Here's how the part is built. I have some questions about the finished solid (model axes, mm). A direction names the side the tool comes from. Coordinates: 2 decimals unless noted, no trailing zeros. Write each loop counter-clockwise with the first axis right and the second up, starting at its lowest first coordinate (ties: lowest second). Pieces come first, ordered by that corner, then holes. Notation, with made-up numbers: (-6.75, 53) -> (15.25, 53) arc R28 cw to (15.25, 92) -> close; hole circle Ø7 at (33.25, -23). An arc over 180 degrees is marked (long way). Use a Markdown table: item, result. Add a question column.
Item 1: On a 3-axis mill with a long thin cutter (end or side, diameter ignored), from which of +Z, -Z, +X, -X, +Y, -Y can I reach the whole of each face in a straight line? I mean faces 1 (the flat face through (0, 5, -12)), 2 (the flat face through (14.625, -3.5, -4)), 3 (the flat face through (0, 4, -26)), 4 (the cylindrical face through (0, -4, 1)). Say none if no direction works.
Item 2: Imagine slicing it at A-A, the plane x = 0. Write out the boundary of the cut face in (y, z), and give its area (3 significant figures).
Item 3: Will these pins go through, and if not, where does the flat tip stop? pin 1 Ø3 at (x, z) = (12, -16.5) entering from +Y; pin 2 Ø1 at (y, z) = (-6, -12) entering from +X (3 decimals); pin 3 Ø3 at (x, z) = (13.5, -14) entering from +Y.
Item 4: If we mould it in two halves opening along X, with no side actions, what happens to faces 5 (the flat face through (1, -5, 0)), 6 (the cylindrical face through (8.285, -2.699, -12.297)), 7 (the flat face through (-8, 2, -12))? For each: pulls with the +X half, pulls with the -X half, needs draft (parallel to the pull), parting line crosses it, or undercut.
Item 5: Imagine slicing it at C-C, the plane z = -4. Count the separate pieces of the cut face and the enclosed holes in it, and give its area (3 significant figures).
Item 6: Imagine slicing it at B-B, the plane x = -11.5. Write out the boundary of the cut face in (y, z), and give its area (3 significant figures).
Item 7: Imagine slicing it at D-D, the plane y = -5.75. Write out the boundary of the cut face in (x, z) (3 decimals).
Item 8: If I drill on line 1 along Y through (x, z) = (9.75, -25.25); line 2 along X through (y, z) = (-4.8, -4) (3 decimals); line 3 along X through (y, z) = (1, -2.25), over which ranges is the centre line in solid material (lowest first)? Write a range as from..to.
```python
from build123d import *

# Parameters (mm, degrees)
EXTRUDE_1_DEPTH          = 2
EXTRUDE_2_DEPTH          = 27
SKETCH_4_R               = 3.227350269
CUT_EXTRUDE_1_DEPTH      = 2
CUT_EXTRUDE_2_DEPTH      = 11
CUT_EXTRUDE_2_DEPTH_BACK = 0.5
CUT_EXTRUDE_3_DEPTH      = 11
CUT_EXTRUDE_3_DEPTH_BACK = 1
SKETCH_8_W               = 12
SKETCH_8_H               = 1
EXTRUDE_3_DEPTH          = 1.6
SKETCH_10_R              = 1.6
CUT_EXTRUDE_4_DEPTH      = 6
SKETCH_11_R              = 1.3
CUT_EXTRUDE_5_DEPTH      = 6.5


with BuildPart() as part:
    # 草图1 → 凸台-拉伸1 (new body)
    with BuildSketch(Plane.XY):
        with BuildLine():
            Line((-9, -3), (-12.875, -3))
            ThreePointArc((-12.875, -3), (-13.582106781, -3.292893219), (-13.875, -4))
            Line((-13.875, -4), (-13.875, -8))
            ThreePointArc((-13.875, -8), (-13.582106781, -8.707106781), (-12.875, -9))
            Line((-12.875, -9), (15, -9))
            ThreePointArc((15, -9), (15.707106781, -8.707106781), (16, -8))
            Line((16, -8), (16, -4))
            ThreePointArc((16, -4), (15.707106781, -3.292893219), (15, -3))
            Line((15, -3), (9, -3))
            ThreePointArc((9, -3), (8.292893219, -2.707106781), (8, -2))
            Line((8, -2), (8, 6))
            ThreePointArc((8, 6), (7.707106781, 6.707106781), (7, 7))
            Line((7, 7), (-7, 7))
            ThreePointArc((-7, 7), (-7.707106781, 6.707106781), (-8, 6))
            Line((-8, 6), (-8, -2))
            ThreePointArc((-8, -2), (-8.292893219, -2.707106781), (-9, -3))
        make_face()
        with BuildLine():
            Line((-4, 5), (4, 5))
            Line((4, 5), (4, 0))
            ThreePointArc((4, 0), (0, -4), (-4, 0))
            Line((-4, 0), (-4, 5))
        make_face(mode=Mode.SUBTRACT)
    extrude(amount=EXTRUDE_1_DEPTH)

    # 草图2 → 凸台-拉伸2 (add)
    with BuildSketch(Plane(origin=(0, 0, 0), x_dir=(-1, 0, 0), z_dir=(0, 0, -1))):
        with BuildLine():
            Line((-6, 4.5), (-6, 5))
            Line((-6, 5), (-5.5, 5))
            Line((-5.5, 5), (5.5, 5))
            Line((5.5, 5), (6, 5))
            Line((6, 5), (6, 4.5))
            Line((6, 4.5), (6, -4.5))
            Line((6, -4.5), (6, -5))
            Line((6, -5), (11.875, -5))
            Line((11.875, -5), (11.875, -7))
            Line((11.875, -7), (-16, -7))
            Line((-16, -7), (-16, -8))
            ThreePointArc((-16, -8), (-15.707106781, -8.707106781), (-15, -9))
            Line((-15, -9), (12.875, -9))
            ThreePointArc((12.875, -9), (13.582106781, -8.707106781), (13.875, -8))
            Line((13.875, -8), (13.875, -4))
            ThreePointArc((13.875, -4), (13.582106781, -3.292893219), (12.875, -3))
            Line((12.875, -3), (9, -3))
            ThreePointArc((9, -3), (8.292893219, -2.707106781), (8, -2))
            Line((8, -2), (8, 6))
            ThreePointArc((8, 6), (7.707106781, 6.707106781), (7, 7))
            Line((7, 7), (-7, 7))
            ThreePointArc((-7, 7), (-7.707106781, 6.707106781), (-8, 6))
            Line((-8, 6), (-8, -2))
            ThreePointArc((-8, -2), (-8.292893219, -2.707106781), (-9, -3))
            Line((-9, -3), (-15, -3))
            ThreePointArc((-15, -3), (-15.707106781, -3.292893219), (-16, -4))
            Line((-16, -4), (-16, -5))
            Line((-16, -5), (-6, -5))
            Line((-6, -5), (-6, -4.5))
            Line((-6, -4.5), (-6, 4.5))
        make_face()
    extrude(amount=EXTRUDE_2_DEPTH)

    # 草图4 → 切除-拉伸1 (cut)
    with BuildSketch(Plane.XZ.offset(9)):
        with Locations((11.625, -15.5)):
            Circle(SKETCH_4_R)
    extrude(amount=-CUT_EXTRUDE_1_DEPTH, mode=Mode.SUBTRACT)

    # 草图5 → 切除-拉伸2 (cut, two sides)
    with BuildSketch(Plane(origin=(0, -3, 0), x_dir=(1, 0, 0), z_dir=(0, 1, 0))) as cut_extrude_2_sk:
        Polygon((11.625, 18.675426481), (8.875, 17.08771324), (8.875, 13.91228676), (11.625, 12.324573519), (14.375, 13.91228676), (14.375, 17.08771324), align=None)
    extrude(amount=CUT_EXTRUDE_2_DEPTH, mode=Mode.SUBTRACT)
    extrude(cut_extrude_2_sk.sketch, amount=-CUT_EXTRUDE_2_DEPTH_BACK, mode=Mode.SUBTRACT)

    # 草图6 → 切除-拉伸3 (cut, two sides)
    with BuildSketch(Plane(origin=(0, -3, 0), x_dir=(1, 0, 0), z_dir=(0, 1, 0))) as cut_extrude_3_sk:
        Polygon((14.625, 2.267949192), (14.625, 5.732050808), (11.625, 7.464101615), (8.625, 5.732050808), (8.625, 2.267949192), (11.625, 0.535898385), align=None)
    extrude(amount=CUT_EXTRUDE_3_DEPTH, mode=Mode.SUBTRACT)
    extrude(cut_extrude_3_sk.sketch, amount=-CUT_EXTRUDE_3_DEPTH_BACK, mode=Mode.SUBTRACT)

    # 草图8 → 凸台-拉伸3 (add)
    with BuildSketch(Plane(origin=(0, 0, -27), x_dir=(-1, 0, 0), z_dir=(0, 0, -1))):
        with Locations((0, 4.5)):
            Rectangle(SKETCH_8_W, SKETCH_8_H)
    extrude(amount=-EXTRUDE_3_DEPTH)

    # 草图10 → 切除-拉伸4 (cut, through all)
    with BuildSketch(Plane(origin=(0, -4, 0), x_dir=(1, 0, 0), z_dir=(0, 1, 0))):
        with Locations((11.625, 4)):
            Circle(SKETCH_10_R)
    extrude(amount=-CUT_EXTRUDE_4_DEPTH, mode=Mode.SUBTRACT)

    # 草图11 → 切除-拉伸5 (cut, through all)
    with BuildSketch(Plane(origin=(0, -3.5, 0), x_dir=(1, 0, 0), z_dir=(0, 1, 0))):
        with Locations((11.678753785, 15.531034762)):
            Circle(SKETCH_11_R)
    extrude(amount=-CUT_EXTRUDE_5_DEPTH, mode=Mode.SUBTRACT)


solid = part.part
```
Ans:
| question | item | result |
|---|---|---|
| 1 | face 1 | none |
| 1 | face 2 | +Y |
| 1 | face 3 | -Z |
| 1 | face 4 | +Z, -Z |
| 2 | outline | (-9, -27) -> (-7, -27) -> (-7, 0) -> (-4, 0) -> (-4, 2) -> (-9, 2) -> close; (4, -27) -> (7, -27) -> (7, 2) -> (5, 2) -> (5, -25.4) -> (4, -25.4) -> close |
| 2 | area | 124 mm^2 |
| 3 | pin 1 | stops at y = -3.5 |
| 3 | pin 2 | stops at x = -11.875 |
| 3 | pin 3 | stops at y = -3 |
| 4 | face 5 | undercut |
| 4 | face 6 | pulls with the +X half |
| 4 | face 7 | pulls with the -X half |
| 5 | separate pieces | 3 |
| 5 | enclosed holes | 0 |
| 5 | area | 147 mm^2 |
| 6 | outline | (-9, -27) -> (-7, -27) -> (-7, 0) -> (-5, 0) -> (-5, -27) -> (-3, -27) -> (-3, 2) -> (-9, 2) -> close |
| 6 | area | 120 mm^2 |
| 7 | outline | (-13.875, -27) -> (-11.875, -27) -> (-11.875, 0) -> (16, 0) -> (16, 2) -> (-13.875, 2) -> close |
| 8 | line 1 | y = -9..-7, -5..-3 |
| 8 | line 2 | x = -13.875..-6, 6..10.025, 13.225..16 |
| 8 | line 3 | x = -8..-6, 6..8 |
